Read the model definition and answer for the solid it produces. Units are mm, in the model's axes. A direction names the side the tool comes from. Give positions to 0.01 mm unless a question says otherwise; leave off trailing zeros. Order: outer loops, then holes, each group sorted by start corner. A loop starts at its lowest first (then second) coordinate and runs counter-clockwise, first axis right, second up. Notation, with made-up numbers: (-30.75, 65) - (2.25, 65) arc R20 ccw to (2.25, 79) - close; hole circle Ø1 at (77, -8.5). An arc over 180 degrees is marked (long way). Write item = value, one per line.
```python
from build123d import *

# Parameters (mm, degrees)
SKETCH1_W               = 8
SKETCH1_H               = 8
BOSS_EXTRUDE1_DEPTH     = 3
CUT_EXTRUDE1_DEPTH      = 12.704699911
CUT_EXTRUDE1_DEPTH_BACK = 12.704699911
CUT_EXTRUDE2_DEPTH      = 11
SKETCH4_R               = 1.75
CUT_EXTRUDE3_DEPTH      = 0.4
SKETCH5_W               = 8
SKETCH5_H               = 1
BOSS_EXTRUDE2_DEPTH     = 2
FILLET1_R               = 4
CUT_EXTRUDE4_DEPTH      = 0.4
CUT_EXTRUDE5_DEPTH      = 0.4


with BuildPart() as part:
    # Sketch1 → Boss-Extrude1 (new body)
    with BuildSketch(Plane(origin=(0, 0, 0), x_dir=(1, 0, 0), z_dir=(0, 1, 0))):
        with Locations((4, 4)):
            Rectangle(SKETCH1_W, SKETCH1_H)
    extrude(amount=BOSS_EXTRUDE1_DEPTH)

    # Sketch2 → Cut-Extrude1 (cut, two sides: drawn at the far end of the back side and taken through both)
    with BuildSketch(Plane.XY.offset(-CUT_EXTRUDE1_DEPTH_BACK)):
        Polygon((0, 0), (0.6, 3), (0, 3), align=None)
        Polygon((8, 0), (7.4, 3), (8, 3), align=None)
    extrude(amount=CUT_EXTRUDE1_DEPTH + CUT_EXTRUDE1_DEPTH_BACK, mode=Mode.SUBTRACT)

    # Sketch3 → Cut-Extrude2 (cut)
    with BuildSketch(Plane(origin=(0, 0, 0), x_dir=(0, 0, -1), z_dir=(1, 0, 0))):
        Polygon((0, 0), (0.6, 3), (0, 3), align=None)
        Polygon((8, 3), (7.4, 3), (8, 0), align=None)
    extrude(amount=CUT_EXTRUDE2_DEPTH, mode=Mode.SUBTRACT)

    # Sketch4 → Cut-Extrude3 (cut)
    with BuildSketch(Plane.XZ):
        with Locations(Location((4, -3.75, 0), (0, 0, 270))):
            Circle(SKETCH4_R)
    extrude(amount=-CUT_EXTRUDE3_DEPTH, mode=Mode.SUBTRACT)

    # Sketch5 → Boss-Extrude2 (add)
    with BuildSketch(Plane.XZ):
        with Locations((4, -7.5)):
            Rectangle(SKETCH5_W, SKETCH5_H)
    extrude(amount=BOSS_EXTRUDE2_DEPTH)

    # Fillet1
    # the kernel refuses this fillet: 4 mm, written as the material it takes off along each edge
    with BuildSketch(Plane(origin=(8, -2, -16.660254038), x_dir=(0, 1, 0), z_dir=(0, 0, 1)), Plane(origin=(0, -2, 1.660254038), x_dir=(0, 1, 0), z_dir=(0, 0, -1))) as fillet1_piece_1:
        with BuildLine():
            CenterArc((4, 3.464101615), FILLET1_R, 180, 60)
            Line((0, 3.464101615), (-0.08, 3.464101615))
            Line((-0.08, 3.464101615), (-0.08, 0))
            Line((-0.08, 0), (0, -0.08))
            ThreePointArc((0, -0.08), (1, -0.08), (1.96, -0.069282032))
            Line((1.96, -0.069282032), (2, 0))
        make_face()
    extrude(amount=18.320508076, mode=Mode.SUBTRACT)

    # Sketch6 → Cut-Extrude4 (cut)
    with BuildSketch(Plane(origin=(0, 3, 0), x_dir=(1, 0, 0), z_dir=(0, 1, 0))):
        Polygon((2.721575188, 1.941169366), (2.721575188, 5.941169366), (5.439523906, 5.941169366), (5.439523906, 5.2745027), (3.490805957, 5.2745027), (3.490805957, 4.300143725), (5.18311365, 4.300143725), (5.18311365, 3.633477059), (3.490805957, 3.633477059), (3.490805957, 1.941169366), align=None)
    extrude(amount=-CUT_EXTRUDE4_DEPTH, mode=Mode.SUBTRACT)

    # Sketch7 → Cut-Extrude5 (cut)
    with BuildSketch(Plane(origin=(0, 3, 0), x_dir=(1, 0, 0), z_dir=(0, 1, 0))):
        Polygon((6.374503362, 0.955347226), (6.374503362, 3.239962611), (7.020657208, 3.239962611), (7.020657208, 2.939962611), (6.720657208, 2.939962611), (6.720657208, 1.255347226), (7.020657208, 1.255347226), (7.020657208, 0.955347226), align=None)
    extrude(amount=-CUT_EXTRUDE5_DEPTH, mode=Mode.SUBTRACT)


solid = part.part
```
1. Section C-C (y = 1.2) is taken. Determine the outline of the cut face in (x, z), and give its area (3 significant figures).
Recorded:
outline = (0.24, -7.76) - (7.76, -7.76) - (7.76, -0.24) - (0.24, -0.24) - close
area = 56.6 mm^2
2. Section A-A (z = -1.75) is taken. Determine the outline of the cut face in (x, y), and give its area (3 significant figures).
Recorded:
outline = (0, 0) - (8, 0) - (7.4, 3) - (6.72, 3) - (6.72, 2.6) - (6.37, 2.6) - (6.37, 3) - (0.6, 3) - close
area = 22.1 mm^2
3. For faces 5 (the face through (3, 0, -2)), 6 (the face through (4, 0.4, -4)), 7 (the face through (6.51, -1.48, -7.51)), determine the directions among +Z, -Z, +X, -X, +Y, -Y from which every point of the face is accessible in a straight line to the end or side of a thin tool.
Recorded:
face_5 = +Z, +X, -X, -Y
face_6 = -Y
face_7 = +Z, -Z, +X, -Y
4. Section D-D (z = -3.75) is taken. Determine the outline of the cut face in (x, y).
Recorded:
outline = (0, 0) - (2.25, 0) - (2.25, 0.4) - (5.75, 0.4) - (5.75, 0) - (8, 0) - (7.4, 3) - (5.18, 3) - (5.18, 2.6) - (2.72, 2.6) - (2.72, 3) - (0.6, 3) - close
5. Section B-B (x = 4) is taken. Determine the outline of the cut face in (y, z).
Recorded:
outline = (-2, -8) - (0, -8) - (3, -7.4) - (3, -5.94) - (2.6, -5.94) - (2.6, -5.27) - (3, -5.27) - (3, -4.3) - (2.6, -4.3) - (2.6, -3.63) - (3, -3.63) - (3, -0.6) - (0, 0) - (0, -2) - (0.4, -2) - (0.4, -5.5) - (0, -5.5) - (0, -7) - (-2, -7) - close
6. Determine the mould class of faces 1 (the face through (2.94, 0.2, -2.36)), 2 (the face through (7.7, 1.5, -4.1)), 3 (the face through (0.3, 1.5, -4.1)), 4 (the face through (4, 3, -5)) for opening direction X: +X half, -X half, draft (parallel to the pull), parting line (faces both ways), or undercut.
Recorded:
face_1 = undercut
face_2 = +X half
face_3 = -X half
face_4 = draft
7. Flat-ended cylindrical pins translate along their axes: pin 1 (2 mm diameter, centred on x = 4.5, z = -2.5, fed in from -Y); pin 2 (4 mm diameter, centred on x = 6.5, z = -5.5, fed in from -Y). Find the tip coordinate at first contact, or state that the pin passes through.
Recorded:
pin_1 = 0
pin_2 = -1.95
8. Straight lines are drawn through the part: L1, parallel to X at y = 0.35, z = -3.75; L2, parallel to Y at x = 5, z = -5.75; L3, parallel to Y at x = 2.5, z = -4. For each, find the intervals that lie inside material, in ascending order. Write a range as [from, to].
Recorded:
L1 = [0.07, 2.25], [5.75, 7.93]
L2 = [0, 2.6]
L3 = [0.4, 3]
